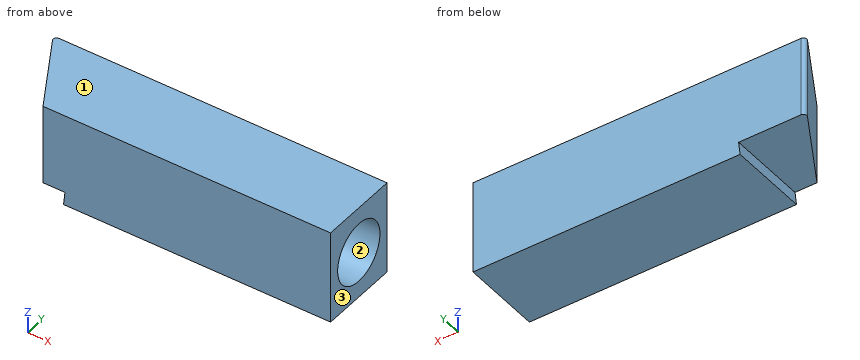
from build123d import *

# Parameters (mm, degrees)
EXTRUDE1_DEPTH     = 14
CUT_EXTRUDE1_DEPTH = 14
FILLET1_R          = 0.5
SKETCH3_R          = 4.5
CUT_EXTRUDE2_DEPTH = 25


with BuildPart() as part:
    # Sketch1 → Extrude1 (new body)
    with BuildSketch(Plane.XY):
        Polygon((-22.646297813, 12), (27.353702187, 12), (27.353702187, 0), (-15.718094583, 0), align=None)
    extrude(amount=EXTRUDE1_DEPTH)

    # Sketch2 → Cut-Extrude1 (cut)
    with BuildSketch(Plane(origin=(0, 12, 0), x_dir=(1, 0, 0), z_dir=(0, 1, 0))):
        Polygon((-22.646297813, -2), (-12.427539106, -2), (-12.646297813, 0), (-22.646297813, 0), align=None)
    extrude(amount=-CUT_EXTRUDE1_DEPTH, mode=Mode.SUBTRACT)

    # Fillet1
    fillet1_edges = [part.edges().sort_by_distance(p)[0] for p in [
        (-22.646297813, 12, 8),
    ]]
    fillet(fillet1_edges, radius=FILLET1_R)

    # Sketch3 → Cut-Extrude2 (cut)
    with BuildSketch(Plane(origin=(27.353702187, 0, 0), x_dir=(0, 0, -1), z_dir=(1, 0, 0))):
        with Locations((-7, 6)):
            Circle(SKETCH3_R)
    extrude(amount=-CUT_EXTRUDE2_DEPTH, mode=Mode.SUBTRACT)


solid = part.part
Verification items for the finished model (mm, model axes). Face numbers are marked on the shaded views. Give positions to 0.01 mm unless a question says otherwise; leave off trailing zeros. Order: outer loops, then holes, each group sorted by start corner. A loop starts at its lowest first (then second) coordinate and runs counter-clockwise, first axis right, second up. Notation, with made-up numbers: M 50,42.5 L 94,42.5 A21 ccw 94,46.5 Z; hole C 18.5,43.5 d9. An arc over 180 degrees is marked long. Use one line per item in the form item = value. Start each with the question number.
Q1. Section check A-A (x = 16). Enter the section's corners in (y, z), then the cut area to 3 significant figures.
Q2. Go/stop test with flat-tipped pins: pin 1 Ø7 at (y, z) = (6, 7) entering from +X; pin 2 Ø3 at (y, z) = (8.5, 6.5) entering from -X; pin 3 Ø1.5 at (y, z) = (4.5, 3) entering from -X. Record where each tip stops, or that it passes through.
Q3. Section check B-B (z = 7). Enter the section's corners in (x, y), then the cut area to 3 significant figures.
Q4. Section check C-C (y = 2.75). Enter the section's corners in (x, z), then the cut area to 3 significant figures.
Q5. Mould release check, pull along Z, two halves, no side actions. Record for the marked faces 1, 2 and 3: +Z half, -Z half, draft (parallel to the pull), parting line (faces both ways), or undercut.
Q6. Section check D-D (x = -14). Enter the section's corners in (y, z).
Q7. Scan lines: line 1 along Y through (x, z) = (11.5, 7); line 2 along Z through (x, y) = (-14, 4.5); line 3 along Y through (x, z) = (18.5, 6). Record each from-to range of solid material in increasing order. Write a range as [from, to].
Evaluation:
q1.outline = M 0,0 L 12,0 L 12,14 L 0,14 Z; hole C 6,7 d9
q1.area = 104 mm2
q2.pin_1 = 2.35
q2.pin_2 = -21.49
q2.pin_3 = -18.75
q3.outline = M -22.21,11.25 L -15.72,0 L 27.35,0 L 27.35,1.5 L 2.35,1.5 L 2.35,10.5 L 27.35,10.5 L 27.35,12 L -21.78,12 A0.5 ccw Z
q3.area = 333 mm2
q4.outline = M -17.31,2 L -12.43,2 L -12.65,0 L 27.35,0 L 27.35,3.89 L 2.35,3.89 L 2.35,10.11 L 27.35,10.11 L 27.35,14 L -17.31,14 Z
q4.area = 460 mm2
q5.face_1 = +Z half
q5.face_2 = undercut
q5.face_3 = draft
q6.outline = M 0,2 L 12,2 L 12,14 L 0,14 Z
q7.line_1 = [0, 1.5], [10.5, 12]
q7.line_2 = [2, 14]
q7.line_3 = [0, 1.61], [10.39, 12]
